Autodesk Fusion 360 part; units mm, degrees
sketch "Esquisse1" plane through (0, 0, 0) normal (0, 1, 0) x (1, 0, 0)
  circle A0 centre (0, 0) radius 5
  dimension "d1" = 10
extrude "Extrusion1" add sketch "Esquisse1" along normal blind 8
sketch "Esquisse2" plane through (0, 8, 0) normal (0, 1, 0) x (-1, 0, 0)
  circle A0 centre (0, 0) radius 5
  circle A1 centre (0, 0) radius 9
  dimension "d4" = 18
extrude "Extrusion2" add sketch "Esquisse2" along normal blind 93 contours A0 | A1
sketch "Esquisse3" plane through (0, 0, 0) normal (0, -1, 0) x (1, 0, 0)
  circle A0 centre (0, 0) radius 5
  circle A1 centre (0, 0) radius 2.5
  dimension "d7" = 5
extrude "Extrusion3" add sketch "Esquisse3" along normal blind 20 contours A1
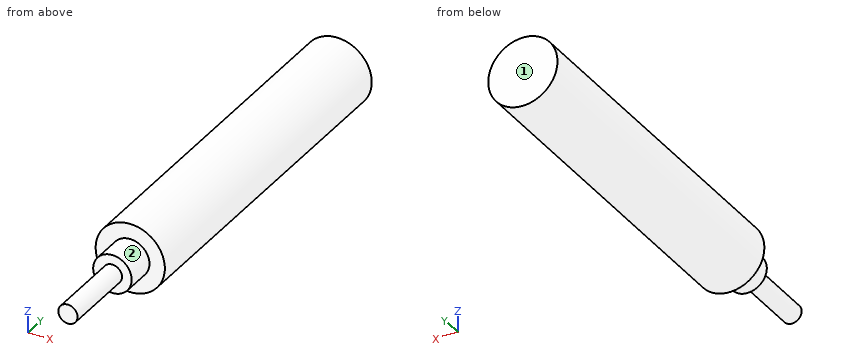
Here's how the part is built. I have some questions about the finished solid (model axes, mm). Face numbers are marked on the shaded views. A direction names the side the tool comes from. Round coordinates to 2 decimals unless told otherwise and drop trailing zeros. Loops run counter-clockwise (first coordinate to the right, second up) from the corner with the lowest first, then second, coordinate; pieces in that order, holes last.
1. Suppose I cut it at A-A, the plane x = 0. Please give me the cut outline in (y, z), and give its area (3 significant figures).
Answers:
outline: (-20, -2.5) - (0, -2.5) - (0, -5) - (8, -5) - (8, -9) - (101, -9) - (101, 9) - (8, 9) - (8, 5) - (0, 5) - (0, 2.5) - (-20, 2.5) - close
area: 1,850 mm2
2. If I drill on probe 1 along Y at (x, z) = (1.5, 8); probe 2 along Y at (x, z) = (-3, 0.5); probe 3 along Z at (x, y) = (-0.25, 47), over which ranges is the centre line in solid material (lowest first)?
Answers:
probe 1: y = 8 to 101
probe 2: y = 0 to 101
probe 3: z = -9 to 9
3. Suppose I cut it at D-D, the plane x = -6.5. Please give me the cut outline in (y, z), and give its area (3 significant figures).
Answers:
outline: (8, -6.22) - (101, -6.22) - (101, 6.22) - (8, 6.22) - close
area: 1,160 mm2
4. Will these pins go through, and if not, where does the flat tip stop? pin 1 (5 mm diameter, centred on x = -1.5, z = -7, fed in from -Y); pin 2 (2 mm diameter, centred on x = -6, y = 70.5, fed in from -Z); pin 3 (1.5 mm diameter, centred on x = 4.5, y = 86.5, fed in from +Z).
Answers:
pin 1: stops at y = 0
pin 2: stops at z = -7.48
pin 3: stops at z = 8.18
5. For the marked faces 1 and 2, which set-ups out of +Z, -Z, +X, -X, +Y, -Y let a thin tool reach every point of the face, with its end or its side?
Answers:
face 1: +Z, -Z, +X, -X, +Y
face 2: -Y
6. Suppose I cut it at C-C, the plane y = 17. Please give me the cut outline in (x, z), and give its area (3 significant figures).
Answers:
outline: circle Ø18 at (0, 0)
area: 254 mm2
7. Suppose I cut it at B-B, the plane z = 0. Please give me the cut outline in (x, y).
Answers:
outline: (-9, 8) - (-5, 8) - (-5, 0) - (-2.5, 0) - (-2.5, -20) - (2.5, -20) - (2.5, 0) - (5, 0) - (5, 8) - (9, 8) - (9, 101) - (-9, 101) - close
